```python
from build123d import *

# Parameters (mm, degrees)
F_1_1_DIAMETER_HOLE1_D = 25.4
CIRPATTERN1_COUNT      = 5
FILLET2_R              = 10.795


with BuildPart() as part:
    # Sketch1 → Revolve1 (revolve)
    with BuildSketch(Plane.XY, mode=Mode.PRIVATE) as revolve1_sk:
        Polygon((87.63, 0), (57.15, 0), (57.15, 5.08), (0, 5.08), (0, 15.24), (57.15, 15.24), (57.15, 31.75), (79.9973, 31.75), (79.9973, 26.035), (87.63, 26.035), align=None)
    revolve(revolve1_sk.sketch.rotate(Axis((0, 5.08, 0), (0, 1, 0)), 90), axis=Axis((0, 5.08, 0), (0, 1, 0)))

    # 1 (1) Diameter Hole1 (through all)
    with Locations(Plane(origin=(0, 15.24, 0), x_dir=(1, 0, 0), z_dir=(0, 1, 0))):
        with Locations((0, 0)):
            Hole(F_1_1_DIAMETER_HOLE1_D / 2)

    # Sketch7 → 3/16 (0.1865) Dowel Hole1 (revolve, cut)
    with BuildSketch(Plane(origin=(0, 31.75, -66.675), x_dir=(0, 0, 1), z_dir=(1, 0, 0))):
        Polygon((0, 0), (0, 14.123168419), (2.36855, 12.7), (2.36855, 0), align=None)
    f_3_16_0_1865_dowel_hole1 = revolve(axis=Axis((0, 38.1, -66.675), (0, -1, 0)), mode=Mode.SUBTRACT)

    # CirPattern1: 3/16 (0.1865) Dowel Hole1 ×5 about axis
    cirpattern1_axis = Axis((0, 0, 0), (0, 1, 0))
    for i in range(1, CIRPATTERN1_COUNT):
        add(f_3_16_0_1865_dowel_hole1.rotate(cirpattern1_axis, i * 360 / CIRPATTERN1_COUNT), mode=Mode.SUBTRACT)

    # Fillet2
    # the kernel refuses this fillet: 10.795 mm, written as the material it adds along each edge
    with BuildSketch(Plane(origin=(0, 5.08, 0), x_dir=(0, 0, -1), z_dir=(1, 0, 0))) as fillet2_piece_1:
        with BuildLine():
            CenterArc((47.99189976, -10.795), FILLET2_R, 31.965718751, 58.034281249)
            Line((47.99189976, 0), (47.99189976, 0.2159))
            Line((47.99189976, 0.2159), (57.15, 0.2159))
            Line((57.15, 0.2159), (57.3659, 0))
            ThreePointArc((57.3659, 0), (57.3659, -2.54), (57.333162005, -4.9657))
            Line((57.333162005, -4.9657), (57.15, -5.08))
        make_face()
    revolve(axis=Axis((0, 5.08, 0), (0, 1, 0)))
    with BuildSketch(Plane(origin=(0, 15.24, 0), x_dir=(0, 0, -1), z_dir=(1, 0, 0))) as fillet2_piece_2:
        with BuildLine():
            CenterArc((57.15 - FILLET2_R, FILLET2_R), FILLET2_R, 270, 90)
            Line((57.15, FILLET2_R), (57.15 + FILLET2_R * 0.02, FILLET2_R))
            Line((57.15 + FILLET2_R * 0.02, FILLET2_R), (57.15 + FILLET2_R * 0.02, -FILLET2_R * 0.02))
            Line((57.15 + FILLET2_R * 0.02, -FILLET2_R * 0.02), (57.15 - FILLET2_R, -FILLET2_R * 0.02))
            Line((57.15 - FILLET2_R, -FILLET2_R * 0.02), (57.15 - FILLET2_R, 0))
        make_face()
    revolve(axis=Axis((0, 15.24, 0), (0, 1, 0)))


solid = part.part
```
Design review of the part built by this model. Coordinates are the model's own, in mm. A direction names the side the tool comes from. Coordinates: 2 decimals unless noted, no trailing zeros. Order: outer loops, then holes, each group sorted by start corner. A loop starts at its lowest first (then second) coordinate and runs counter-clockwise, first axis right, second up.
1) Mouldability with a two-part tool opening along X and no side actions: class faces 4 (the cylindrical face through (-2.513, 28.933, 57.095)), 5 (the cylindrical face through (78.095, 28.852, 17.342)), 6 (the flat face through (39, 26.035, 71)) as +X half, -X half, draft (parallel to the pull), parting line (faces both ways), or undercut.
2) Take a section at B-B, the plane y = 24. Give the boundary of the cut face in (x, z) (3 decimals).
3) For faces 1 (the cylindrical face through (64.61, 25.49, -18.56)), 2 (the flat face through (-54.5, 31.75, -18.9)), 3 (the flat face through (10, 5.08, -10)), list the 3-axis set-ups (+Z, -Z, +X, -X, +Y, -Y) from which the entire face can be reached by the end or side of a thin tool; tool diameter is ignored.
4) Wall thickness on line 1 along Y through (x, z) = (55.5, 65.5) (3 decimals); line 2 along Y through (x, z) = (43.5, 12); line 3 along X through (y, z) = (3.5, -11): over which ranges is each line inside the solid? List them lowest first.
5) Clearance check with flat-ended pins moving along their axes: pin 1 (4 mm diameter, centred on x = 14, z = -31.5, fed in from -Y); pin 2 (4.5 mm diameter, centred on x = 63.41, z = -20.6, fed in from +Y); pin 3 (8 mm diameter, centred on x = -60.5, y = 26.5, fed in from +Z). State where each tip first meets the part, or that it passes through.
6) Take a section at C-C, the plane x = 74. Give the boundary of the cut face in (y, z) (3 decimals).
7) Take a section at D-D, the plane y = 12. Give the boundary of the cut face in (x, z), and give its area (3 significant figures).
8) Take a section at A-A, the plane z = 0. Give the boundary of the cut face in (x, y) (3 decimals).
Returned:
1. face 4: undercut
1. face 5: parting line
1. face 6: draft
2. outline: circle Ø175.26 at (0, 0); hole circle Ø4.737 at (-63.412, -20.604); hole circle Ø113.913 at (0, 0); hole circle Ø4.737 at (-39.191, 53.941); hole circle Ø4.737 at (0, -66.675); hole circle Ø4.737 at (39.191, 53.941); hole circle Ø4.737 at (63.412, -20.604)
3. face 1: +Y
3. face 2: +Z, -Z, +X, -X, +Y
3. face 3: -Y
4. line 1: y = 0 to 26.035
4. line 2: y = 5.08 to 15.24
4. line 3: x = -86.94 to -52.47, 52.47 to 86.94
5. pin 1: stops at y = 5.08
5. pin 2: stops at y = 18.98
5. pin 3: stops at z = 66.96
6. outline: (0, -46.936) - (26.035, -46.936) - (26.035, -30.39) - (31.75, -30.39) - (31.75, 30.39) - (26.035, 30.39) - (26.035, 46.936) - (0, 46.936) - close
7. outline: circle Ø175.26 at (0, 0); hole circle Ø25.4 at (0, 0)
7. area: 23,600 mm2
8. outline: (-87.63, 0) - (-57.15, 0) arc R10.795 cw to (-47.992, 5.08) - (-12.7, 5.08) - (-12.7, 15.24) - (-46.355, 15.24) arc R10.795 cw to (-57.15, 26.035) - (-57.15, 31.75) - (-79.997, 31.75) - (-79.997, 26.035) - (-87.63, 26.035) - close; (12.7, 5.08) - (47.992, 5.08) arc R10.795 cw to (57.15, 0) - (87.63, 0) - (87.63, 26.035) - (79.997, 26.035) - (79.997, 31.75) - (57.15, 31.75) - (57.15, 26.035) arc R10.795 cw to (46.355, 15.24) - (12.7, 15.24) - close
